Read the model definition and answer for the solid it produces. Units are mm, in the model's axes. A direction names the side the tool comes from. Coordinates: 2 decimals unless noted, no trailing zeros. Write each loop counter-clockwise with the first axis right and the second up, starting at its lowest first coordinate (ties: lowest second). Pieces come first, ordered by that corner, then holes. Notation, with made-up numbers: (-26.5, 46) -> (-15.5, 46) arc R35 cw to (-15.5, 82) -> close; hole circle Ø1 at (-29, -18.5). An arc over 180 degrees is marked (long way). Answer as a JSON object with one key per item and string values. Group by question number.
(1) For a pull along X with two mould halves and no side action, classify faces 1 (the face through (96, -1, 2)), 2 (the face through (-1, -58, 2)), 3 (the face through (-82.689, 43.325, 6.465)), 4 (the face through (-13.1, 1.09, 4.56)) as +X half, -X half, draft (parallel to the pull), parting line (faces both ways), or undercut.
(2) Find section A-A (z = 7). Count the separate pieces of the cut face and the enclosed holes in it, then the cut area to 3 significant figures.
(3) Which of the six approach directions +Z, -Z, +X, -X, +Y, -Y give full straight-line access (tool end or side, diameter ignored) to faces 5 (the face through (0, 56, 6)), 6 (the face through (13.8, -15.7, 4)), 7 (the face through (83, 44, 6))?
(4) Find section D-D (x = 52). Give the vertices of the cut face in (y, z).
(5) Flat-ended cylindrical pins translate along their axes: P1, Ø1.5, axis at x = 5.5, z = 7.5, coming from the +Y side; P2, Ø1.5, axis at y = -42, z = 7, coming from the -X side. Find the tip coordinate at first contact, or state that the pin passes through.
(6) Find section C-C (x = -11). Give the vertices of the cut face in (y, z).
(7) Find section B-B (y = 1). Give the vertices of the cut face in (x, z), then the cut area to 3 significant figures.
(8) Straight lines are drawn through the part: L1, parallel to Y at x = -4.5, z = 6.5; L2, parallel to Y at x = -11, z = 7; L3, parallel to Y at x = -84, z = 1.55. For each, find the intervals that lie inside material, in ascending order.
from build123d import *

# Parameters (mm, degrees)
SKETCH_W        = 192
SKETCH_H        = 116
PAD_DEPTH       = 4
SKETCH001_W     = 160
SKETCH001_H     = 40
PAD001_DEPTH    = 5
SKETCH002_R     = 1.4
POCKET_DEPTH    = 9.001
PAD002_DEPTH    = 5
SKETCH004_R     = 1.9
SKETCH004_R_2   = 2.1
POCKET001_DEPTH = 9.001


with BuildPart() as part:
    # Sketch → Pad (new body)
    with BuildSketch(Plane.XY):
        Rectangle(SKETCH_W, SKETCH_H)
    extrude(amount=PAD_DEPTH)

    # Sketch001 (on Face6 of Pad) → Pad001 (join)
    with BuildSketch(Plane.XY.offset(4)):
        with Locations((-9, -36)):
            Rectangle(SKETCH001_W, SKETCH001_H)
        with BuildLine():
            Line((69, -18), (69, -54))
            Line((69, -54), (61.5, -54))
            Line((61.5, -51), (61.5, -54))
            ThreePointArc((61.5, -51), (59, -48.5), (56.5, -51))
            Line((56.5, -51), (56.5, -54))
            Line((56.5, -54), (-87, -54))
            Line((-87, -54), (-87, -18))
            Line((-59.5, -18), (-87, -18))
            Line((-59.5, -18), (-59.5, -21))
            ThreePointArc((-59.5, -21), (-57, -23.5), (-54.5, -21))
            Line((-54.5, -21), (-54.5, -18))
            Line((-54.5, -18), (69, -18))
        make_face(mode=Mode.SUBTRACT)
    extrude(amount=PAD001_DEPTH)

    # Sketch002 (on Face11 of Pad001) → Pocket (cut, through all)
    with BuildSketch(Plane.XY.offset(9)):
        with Locations((-57, -21)):
            Circle(SKETCH002_R)
        with Locations((59, -51)):
            Circle(SKETCH002_R)
    extrude(amount=-POCKET_DEPTH, mode=Mode.SUBTRACT)

    # Sketch003 (on Face5 of Pocket) → Pad002 (join)
    with BuildSketch(Plane.XY.offset(4)):
        Polygon((-69, 56), (71, 56), (96, 31), (96, 11), (71, -14), (-69, -14), (-96, 11), (-96, 31), align=None)
    extrude(amount=PAD002_DEPTH)

    # Sketch004 (on Face22 of Pad002) → Pocket001 (cut, through all)
    with BuildSketch(Plane.XY.offset(9)):
        with Locations((-84, 48)):
            Circle(SKETCH004_R)
        with Locations((-84, -48)):
            Circle(SKETCH004_R)
        with Locations((84, -48)):
            Circle(SKETCH004_R)
        with Locations((84, 48)):
            Circle(SKETCH004_R)
        with Locations((-57, 41)):
            Circle(SKETCH004_R_2)
        with Locations((-11, 41)):
            Circle(SKETCH004_R_2)
        with Locations((-57, 1)):
            Circle(SKETCH004_R_2)
        with Locations((-11, 1)):
            Circle(SKETCH004_R_2)
        with Locations((13, 41)):
            Circle(SKETCH004_R_2)
        with Locations((59, 41)):
            Circle(SKETCH004_R_2)
        with Locations((59, 1)):
            Circle(SKETCH004_R_2)
        with Locations((13, 1)):
            Circle(SKETCH004_R_2)
    extrude(amount=-POCKET001_DEPTH, mode=Mode.SUBTRACT)


solid = part.part
Results below:
{
 "1": {"face 1": "+X half", "face 2": "draft", "face 3": "-X half", "face 4": "undercut"},
 "2": {"separate pieces": "2", "enclosed holes": "11", "area": "12,900 mm2"},
 "3": {"face 5": "+Z, +X, -X, +Y", "face 6": "+Z", "face 7": "+Z, +X, +Y"},
 "4": {"outline": "(-58, 0) -> (58, 0) -> (58, 4) -> (56, 4) -> (56, 9) -> (-14, 9) -> (-14, 4) -> (-16, 4) -> (-16, 9) -> (-18, 9) -> (-18, 4) -> (-54, 4) -> (-54, 9) -> (-56, 9) -> (-56, 4) -> (-58, 4) -> close"},
 "5": {"P1": "stops at y = 56", "P2": "stops at x = -89"},
 "6": {"outline": "(-58, 0) -> (-1.1, 0) -> (-1.1, 9) -> (-14, 9) -> (-14, 4) -> (-16, 4) -> (-16, 9) -> (-18, 9) -> (-18, 4) -> (-54, 4) -> (-54, 9) -> (-56, 9) -> (-56, 4) -> (-58, 4) -> close; (3.1, 0) -> (38.9, 0) -> (38.9, 9) -> (3.1, 9) -> close; (43.1, 0) -> (58, 0) -> (58, 4) -> (56, 4) -> (56, 9) -> (43.1, 9) -> close"},
 "7": {"outline": "(-96, 0) -> (-59.1, 0) -> (-59.1, 9) -> (-85.2, 9) -> (-85.2, 4) -> (-96, 4) -> close; (-54.9, 0) -> (-13.1, 0) -> (-13.1, 9) -> (-54.9, 9) -> close; (-8.9, 0) -> (10.9, 0) -> (10.9, 9) -> (-8.9, 9) -> close; (15.1, 0) -> (56.9, 0) -> (56.9, 9) -> (15.1, 9) -> close; (61.1, 0) -> (96, 0) -> (96, 4) -> (86, 4) -> (86, 9) -> (61.1, 9) -> close", "area": "1,470 mm2"},
 "8": {"L1": "y = -56 to -54, -18 to -16, -14 to 56", "L2": "y = -56 to -54, -18 to -16, -14 to -1.1, 3.1 to 38.9, 43.1 to 56", "L3": "y = -58 to -49.9, -46.1 to 46.1, 49.9 to 58"}
}
